from build123d import *

# Parameters (mm, degrees)
F0_W      = 127
F0_H      = 25.4
F1_DEPTH  = 152.4
F2_W      = 98.3371436596
F2_H      = 15.5014246702
F3_DEPTH  = 152.401
F5_DEPTH  = 25.4
F6_R      = 6.8113689933
F7_DEPTH  = 127.001
F10_R     = 7.917856488
F11_DEPTH = 127.001
F12_W     = 98.2769206166
F12_H     = 31.2483850867
F13_DEPTH = 25.401
F14_W     = 98.0260297656
F14_H     = 35.063225776
F15_DEPTH = 25.401
F16_W     = 30.4847359657
F16_H     = 88.5739065707
F17_DEPTH = 25.401


with BuildPart() as f1:
    # F0 (on Right) → F1 (new body)
    with BuildSketch(Plane.YZ):
        with Locations((7.3526296653, 12.7)):
            Rectangle(F0_W, F0_H)
    extrude(amount=F1_DEPTH)

    # F2 (on face) → F3 (cut, through all)
    with BuildSketch(Plane.YZ.offset(152.4)):
        with Locations((7.7507048845, 7.7507123351)):
            Rectangle(F2_W, F2_H)
    extrude(amount=-F3_DEPTH, mode=Mode.SUBTRACT)

    # F4 (on face) → F5 (join)
    with BuildSketch(Plane.YZ.offset(152.4)):
        Polygon((70.8526296653, 25.4), (-56.1473703347, 25.4), (-56.1473703347, 0), (-41.4178669453, 0), (-41.4178669453, 15.5014246702), (56.9192767143, 15.5014246702), (56.9192767143, 0), (70.8526296653, 0), align=None)
    extrude(amount=F5_DEPTH)

    # F6 (on face) → F7 (cut, through all)
    with BuildSketch(Plane(origin=(0, 70.8526296653, 0), x_dir=(-1, 0, 0), z_dir=(0, 1, 0))):
        with Locations((-166.326135397, 16.0321518779)):
            Circle(F6_R)
    extrude(amount=-F7_DEPTH, mode=Mode.SUBTRACT)

    # F10 (on face) → F11 (cut, through all)
    with BuildSketch(Plane(origin=(0, 70.8526296653, 0), x_dir=(-1, 0, 0), z_dir=(0, 1, 0))):
        with Locations((-19.1903246846, 13.7839203013)):
            Circle(F10_R)
    extrude(amount=-F11_DEPTH, mode=Mode.SUBTRACT)

    # F12 (on face) → F13 (cut, through all)
    with BuildSketch(Plane.XY.offset(25.4)):
        with Locations((49.1384603083, -28.1473351642)):
            Rectangle(F12_W, F12_H)
    extrude(amount=-F13_DEPTH, mode=Mode.SUBTRACT)

    # F14 (on face) → F15 (cut, through all)
    with BuildSketch(Plane.XY.offset(25.4)):
        with Locations((49.0130148828, 36.8879642338)):
            Rectangle(F14_W, F14_H)
    extrude(amount=-F15_DEPTH, mode=Mode.SUBTRACT)

    # F16 (on face) → F17 (cut, through all)
    with BuildSketch(Plane.XY.offset(25.4)):
        with Locations((147.2032368183, 6.8099442869)):
            Rectangle(F16_W, F16_H)
    extrude(amount=-F17_DEPTH, mode=Mode.SUBTRACT)


solid = f1.part
Source: CAD feature listing. Evaluate the final solid. Frame: model axes, mm. A direction names the side the tool comes from. Coordinates: 2 decimals unless noted, no trailing zeros. Loops run counter-clockwise (first coordinate to the right, second up) from the corner with the lowest first, then second, coordinate; pieces in that order, holes last. Notation, with made-up numbers: (-31, 5) - (-27, 5) arc R9 cw to (-27, 9) - close; hole circle Ø6 at (40, 69.5). An arc over 180 degrees is marked (long way). One line per item, written item: value. Start each with the question number.
1. Ray query, L1, parallel to Y at x = 27.5, z = 17.5; L2, parallel to Y at x = 140, z = 4.75; L3, parallel to Y at x = 157, z = 19.5. Return the intervals inside material, ascending.
2. Contact query for flat-ended pins moving along their axis: P1, Ø3.5, axis at x = 174.5, y = 11, coming from the -Z side; P2, Ø12.5, axis at y = -25.5, z = 13.5, coming from the -X side; P3, Ø3, axis at y = 31, z = 22, coming from the -X side; P4, Ø10, axis at x = 36.5, y = 48, coming from the +Z side. Output: stop coordinate, or through.
3. Section D-D (y = -20). Return the cut outline in (x, z).
4. Set-up query: faces 1 (the flat face through (98.026, 37, 21)), 2 (the cylindrical face through (19, 3.6, 21.7)), 3 (the cylindrical face through (14.93, 62.75, 20.46)), 4 (the flat face through (137, -41.418, 8)), 5 (the flat face through (147, -37.477, 21)). Return all of +Z, -Z, +X, -X, +Y, -Y with unobstructed straight access to the full face (end or side cutting, diameter ignored); none if empty.
5. Section C-C (z = 2.75). Return the cut outline in (x, y).
6. Section A-A (y = 27). Return the cut outline in (x, z), and give its area (3 significant figures).
7. Mould query, pull axis Z, two halves, no side actions, for faces 6 (the cylindrical face through (171.346, 8.242, 20.636)), 7 (the flat face through (92, 7, 15.501)), 8 (the flat face through (162.446, 6, 24)). Classes: pulls with the +Z half, pulls with the -Z half, needs draft (parallel to the pull), parting line crosses it, or undercut.
8. Section B-B (x = 32.5). Return the cut outline in (y, z), and give its area (3 significant figures).
Verdict:
1. L1: y = -56.15 to -43.77, -12.52 to 19.36, 54.42 to 70.85
1. L2: y = -56.15 to -41.42, 56.92 to 70.85
1. L3: y = -56.15 to -37.48, 51.1 to 70.85
2. P1: stops at z = 15.5
2. P2: stops at x = 98.28
2. P3: stops at x = 98.03
2. P4: passes through
3. outline: (98.28, 15.5) - (131.96, 15.5) - (131.96, 25.4) - (98.28, 25.4) - close; (162.45, 21.63) arc R6.81 cw to (173.12, 15.5) - (177.8, 15.5) - (177.8, 25.4) - (162.45, 25.4) - close
4. face 1: +Z, -Z, -X
4. face 2: -Z, +Y, -Y
4. face 3: +Y, -Y
4. face 4: -Z, +X, -X
4. face 5: +Z, -Z
5. outline: (0, -56.15) - (177.8, -56.15) - (177.8, -41.42) - (98.28, -41.42) - (98.28, -43.77) - (0, -43.77) - close; (0, 56.92) - (177.8, 56.92) - (177.8, 70.85) - (0, 70.85) - close
6. outline: (98.03, 15.5) - (131.96, 15.5) - (131.96, 25.4) - (98.03, 25.4) - close; (162.45, 21.63) arc R6.81 cw to (173.12, 15.5) - (177.8, 15.5) - (177.8, 25.4) - (162.45, 25.4) - close
6. area: 421 mm2
7. face 6: undercut
7. face 7: pulls with the -Z half
7. face 8: needs draft
8. outline: (-56.15, 0) - (-43.77, 0) - (-43.77, 25.4) - (-56.15, 25.4) - close; (-12.52, 15.5) - (19.36, 15.5) - (19.36, 25.4) - (-12.52, 25.4) - close; (54.42, 15.5) - (56.92, 15.5) - (56.92, 0) - (70.85, 0) - (70.85, 25.4) - (54.42, 25.4) - close
8. area: 1,010 mm2
